The figure shows three views and two pictorial views of one solid part (mm, origin at its lowest corner). Answer the questions. A direction names the side the tool comes from. Give positions to 0.01 mm unless a question says otherwise; leave off trailing zeros. Write each loop counter-clockwise with the first axis right and the second up, starting at its lowest first coordinate (ties: lowest second). Pieces come first, ordered by that corner, then holes. Notation, with made-up numbers: (45, 71) - (102, 71) arc R33 cw to (102, 103) - close; hole circle Ø9 at (11.5, 38.5). An arc over 180 degrees is marked (long way). Use a Markdown table: item, result. Add a question column.
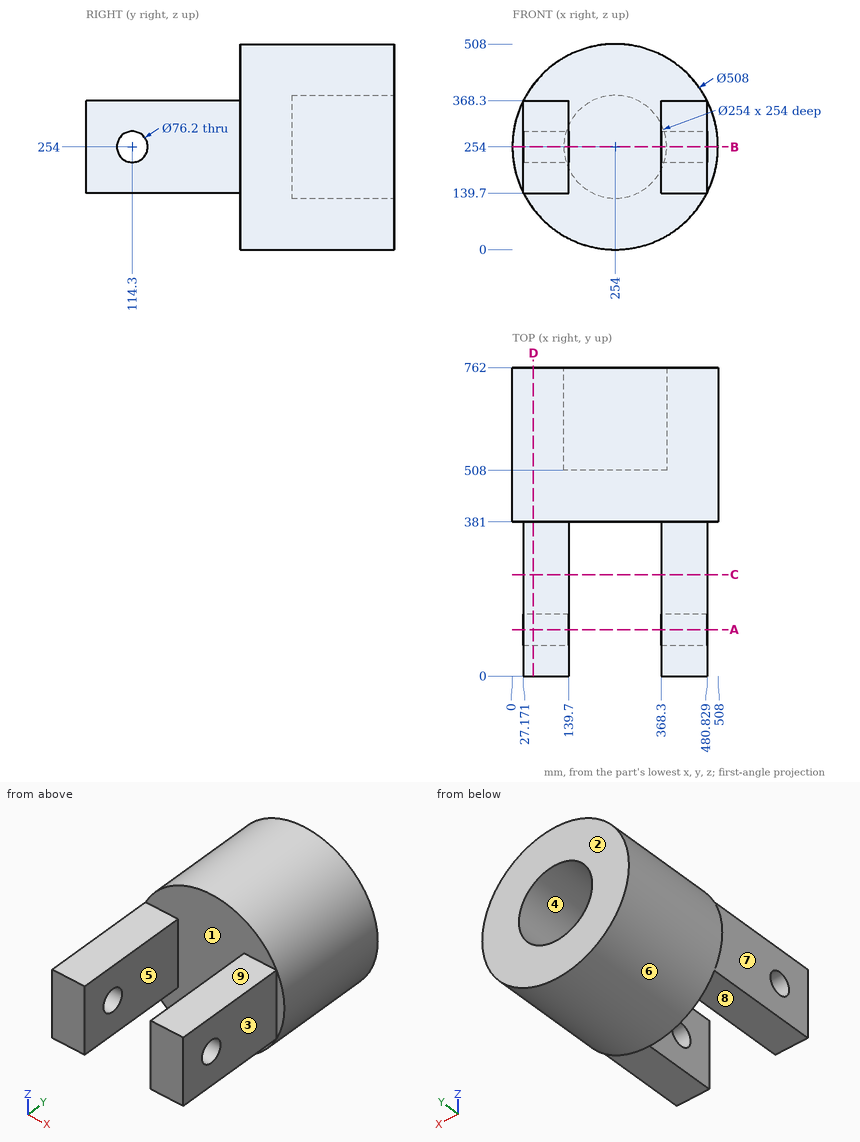
1. The part is cut by section B-B (z = 254). Give the vertices of the cut face in (x, y).
2. The part is cut by section C-C (y = 250.5). Give the vertices of the cut face in (x, z).
3. Consider L1, parallel to Z at x = 56.5, y = 114.3; L2, parallel to X at y = 287.5, z = 275; L3, parallel to X at y = 623, z = 253.5. Determine where each line is inside the solid, lowest interval first. Write a range as [from, to].
4. Given P1, Ø5, axis at x = 143, z = 452.5, coming from the -Y side; P2, Ø12, axis at y = 287, z = 362.5, coming from the -X side, each flat-ended and moving along its own axis, determine where each tip first touches the part or whether it passes through.
5. The part is cut by section A-A (y = 114.3). Give the vertices of the cut face in (x, z), and give its area (3 significant figures).
6. The part is cut by section D-D (x = 52). Give the vertices of the cut face in (y, z).
7. For a pull along X with two mould halves and no side action, classify the marked faces 1, 2, 3 and 4 as released by +X, released by -X, zero draft, split by the parting line, or undercut.
8. Which of the six approach directions +Z, -Z, +X, -X, +Y, -Y give full straight-line access (tool end or side, diameter ignored) to the marked faces 5, 6, 7, 8 and 9?
Check values:
| question | item | result |
|---|---|---|
| 1 | outline | (0, 381) - (27.17, 381) - (27.17, 152.4) - (139.7, 152.4) - (139.7, 381) - (368.3, 381) - (368.3, 152.4) - (480.83, 152.4) - (480.83, 381) - (508, 381) - (508, 762) - (381, 762) - (381, 508) - (127, 508) - (127, 762) - (0, 762) - close; (27.17, 0) - (139.7, 0) - (139.7, 76.2) - (27.17, 76.2) - close; (368.3, 0) - (480.83, 0) - (480.83, 76.2) - (368.3, 76.2) - close |
| 2 | outline | (27.17, 139.7) - (139.7, 139.7) - (139.7, 368.3) - (27.17, 368.3) - close; (368.3, 139.7) - (480.83, 139.7) - (480.83, 368.3) - (368.3, 368.3) - close |
| 3 | L1 | z = [139.7, 215.9], [292.1, 368.3] |
| 3 | L2 | x = [27.17, 139.7], [368.3, 480.83] |
| 3 | L3 | x = [0, 127], [381, 508] |
| 4 | P1 | stops at y = 381 |
| 4 | P2 | stops at x = 27.17 |
| 5 | outline | (27.17, 139.7) - (139.7, 139.7) - (139.7, 215.9) - (27.17, 215.9) - close; (27.17, 292.1) - (139.7, 292.1) - (139.7, 368.3) - (27.17, 368.3) - close; (368.3, 139.7) - (480.83, 139.7) - (480.83, 215.9) - (368.3, 215.9) - close; (368.3, 292.1) - (480.83, 292.1) - (480.83, 368.3) - (368.3, 368.3) - close |
| 5 | area | 34,300 mm2 |
| 6 | outline | (0, 139.7) - (381, 139.7) - (381, 100.01) - (762, 100.01) - (762, 407.99) - (381, 407.99) - (381, 368.3) - (0, 368.3) - close; hole circle Ø76.2 at (114.3, 254) |
| 7 | face 1 | undercut |
| 7 | face 2 | zero draft |
| 7 | face 3 | released by +X |
| 7 | face 4 | undercut |
| 8 | face 5 | +Z, -Z, -Y |
| 8 | face 6 | +Y, -Y |
| 8 | face 7 | +Z, -Z, -X, -Y |
| 8 | face 8 | -Z, +X, -X, -Y |
| 8 | face 9 | +Z, +X, -X, -Y |
